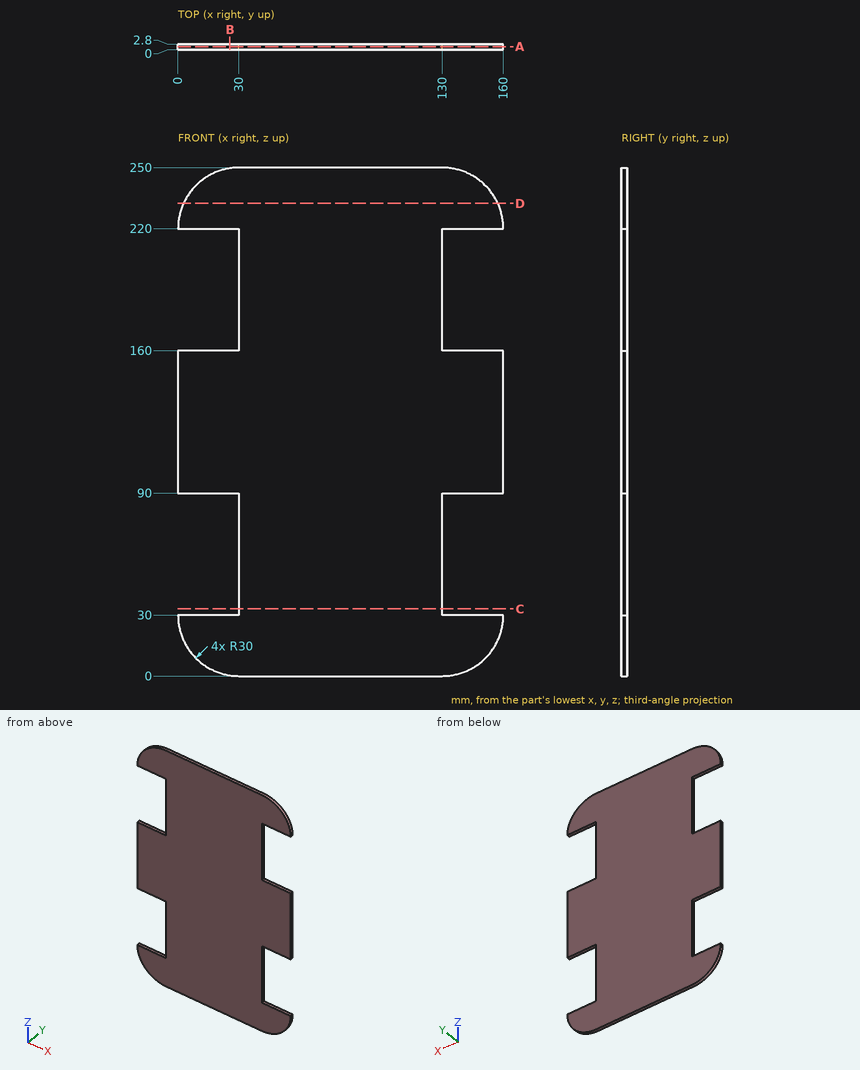
Job drawing, mm, ordinate dimensions from the low corner. One solid piece. Round coordinates to 2 decimals unless told otherwise and drop trailing zeros. Loops run counter-clockwise (first coordinate to the right, second up) from the corner with the lowest first, then second, coordinate; pieces in that order, holes last.
(1) Cut at B-B (x = 25.5). Give the cut face in (y, z), plus the area to 3 significant figures.
(2) Cut at A-A (y = 1.45). Give the cut face in (x, z), plus the area to 3 significant figures.
(3) Cut at C-C (z = 33). Give the cut face in (x, y).
(4) Cut at D-D (z = 232.5). Give the cut face in (x, y), plus the area to 3 significant figures.
(5) Wall check: line 1 along Z through (x, y) = (9, 2.7); line 2 along Z through (x, y) = (26.5, 1.55); line 3 along X through (y, z) = (1.45, 192.5). Give the ranges that are in metal, low to high.
(6) Drop flat-ended pins along their axis: pin 1 (1.4 mm diameter, centred on y = 1, z = 178.5, fed in from +X); pin 2 (0.8 mm diameter, centred on x = 151, y = 1, fed in from -Z); pin 3 (1.4 mm diameter, centred on x = 142, y = 1, fed in from -Z); pin 4 (1.5 mm diameter, centred on x = 99.5, z = 220.5, fed in from -Y). Give the stop position or say it passes through.
Findings below:
1. outline: (0, 0.34) - (2.8, 0.34) - (2.8, 30) - (0, 30) - close; (0, 90) - (2.8, 90) - (2.8, 160) - (0, 160) - close; (0, 220) - (2.8, 220) - (2.8, 249.66) - (0, 249.66) - close
1. area: 362 mm2
2. outline: (0, 30) arc R30 ccw to (30, 0) - (130, 0) arc R30 ccw to (160, 30) - (130, 30) - (130, 90) - (160, 90) - (160, 160) - (130, 160) - (130, 220) - (160, 220) arc R30 ccw to (130, 250) - (30, 250) arc R30 ccw to (0, 220) - (30, 220) - (30, 160) - (0, 160) - (0, 90) - (30, 90) - (30, 30) - close
2. area: 32,000 mm2
3. outline: (30, 0) - (130, 0) - (130, 2.8) - (30, 2.8) - close
4. outline: (2.73, 0) - (157.27, 0) - (157.27, 2.8) - (2.73, 2.8) - close
4. area: 433 mm2
5. line 1: z = 8.58 to 30, 90 to 160, 220 to 241.42
5. line 2: z = 0.2 to 30, 90 to 160, 220 to 249.8
5. line 3: x = 30 to 130
6. pin 1: stops at x = 130
6. pin 2: stops at z = 8.19
6. pin 3: stops at z = 2.21
6. pin 4: stops at y = 0
